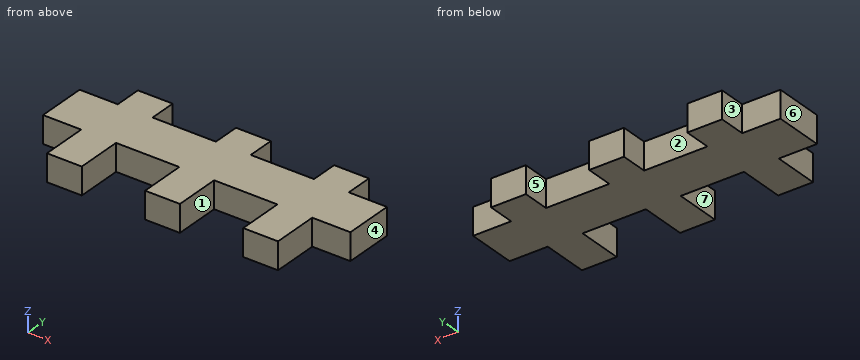
from build123d import *

# Parameters (mm, degrees)
SKETCH1_W           = 4
SKETCH1_H           = 3.175
SKETCH1_W_2         = 42.3
SKETCH1_H_2         = 5.7
SKETCH1_H_3         = 2.225
BOSS_EXTRUDE1_DEPTH = 3.175
CUT_EXTRUDE2_DEPTH  = 23.175
BOSS_EXTRUDE2_DEPTH = 3.175


with BuildPart() as part:
    # Sketch1 → Boss-Extrude1 (new body)
    with BuildSketch(Plane.XY):
        with Locations((-11.5, -1.5875)):
            Rectangle(SKETCH1_W, SKETCH1_H)
        with Locations((-11.5, 7.2875)):
            Rectangle(SKETCH1_W, SKETCH1_H)
        with Locations((0, 7.2875)):
            Rectangle(SKETCH1_W, SKETCH1_H)
        with Locations((0, -1.5875)):
            Rectangle(SKETCH1_W, SKETCH1_H)
        with Locations((11.5, 7.2875)):
            Rectangle(SKETCH1_W, SKETCH1_H)
        with Locations((11.5, -1.5875)):
            Rectangle(SKETCH1_W, SKETCH1_H)
        with Locations((0, 2.85)):
            Rectangle(SKETCH1_W_2, SKETCH1_H_2)
        with Locations((-11.5, -4.2875)):
            Rectangle(SKETCH1_W, SKETCH1_H_3)
        with Locations((0, -4.2875)):
            Rectangle(SKETCH1_W, SKETCH1_H_3)
        with Locations((11.5, -4.2875)):
            Rectangle(SKETCH1_W, SKETCH1_H_3)
    extrude(amount=BOSS_EXTRUDE1_DEPTH)

    # Sketch2 → Cut-Extrude2 (cut)
    with BuildSketch(Plane(origin=(0, 5.7, 0), x_dir=(1, 0, 0), z_dir=(0, 1, 0))):
        Polygon((-17.975, 0), (-21.15, 0), (-21.15, -3.175), align=None)
        Polygon((-17.975, -3.175), (-17.975, 0), (-21.15, -3.175), align=None)
        Polygon((21.15, -3.175), (17.975, -3.175), (17.975, 0), align=None)
        Polygon((21.15, -3.175), (17.975, 0), (21.15, 0), align=None)
    extrude(amount=-CUT_EXTRUDE2_DEPTH, mode=Mode.SUBTRACT)

    # Sketch3 → Boss-Extrude2 (add)
    with BuildSketch(Plane.XY.offset(3.175)):
        Polygon((-13.54064, -5.44064), (-9.45936, -5.44064), (-9.45936, -0.04064), (-2.04064, -0.04064), (-2.04064, -5.44064), (2.04064, -5.44064), (2.04064, -0.04064), (9.45936, -0.04064), (9.45936, -5.44064), (13.54064, -5.44064), (13.54064, -0.04064), (18.01564, -0.04064), (18.01564, 5.74064), (13.54064, 5.74064), (13.54064, 8.91564), (9.45936, 8.91564), (9.45936, 5.74064), (2.04064, 5.74064), (2.04064, 8.91564), (-2.04064, 8.91564), (-2.04064, 5.74064), (-9.45936, 5.74064), (-9.45936, 8.91564), (-13.54064, 8.91564), (-13.54064, 5.74064), (-18.01564, 5.74064), (-18.01564, -0.04064), (-13.54064, -0.04064), align=None)
    extrude(amount=-BOSS_EXTRUDE2_DEPTH)


solid = part.part
Read the model definition and answer for the solid it produces. Units are mm, in the model's axes. Face numbers are marked on the shaded views. A direction names the side the tool comes from. Round coordinates to 2 decimals unless told otherwise and drop trailing zeros. Write each loop counter-clockwise with the first axis right and the second up, starting at its lowest first coordinate (ties: lowest second). Pieces come first, ordered by that corner, then holes. Notation, with made-up numbers: (-6, 27.5) - (19, 27.5) arc R26 cw to (19, 48.5) - close; hole circle Ø4 at (48, 15). An arc over 180 degrees is marked (long way). Use a Markdown table: item, result.
(1) Each of these flat-tipped pins is pushed along its axis until it touches: pin 1 Ø1 at (x, z) = (7.5, 1) entering from -Y; pin 2 Ø1.6 at (y, z) = (-2.5, 2.5) entering from -X; pin 3 Ø1 at (y, z) = (-3, 2.5) entering from +X; pin 4 Ø2 at (x, y) = (12.5, -3) entering from -Z. Where does it stop, or does it pass through?
Reported:
| item | result |
|---|---|
| pin 1 | y = -0.04 |
| pin 2 | x = -13.54 |
| pin 3 | x = 13.54 |
| pin 4 | z = 0 |
(2) The mould has two halves that part along X. Classify the marked faces 4, 5, 6 and 7: released by +X, released by -X, zero draft, split by the parting line, or undercut.
Reported:
| item | result |
|---|---|
| face 4 | released by +X |
| face 5 | undercut |
| face 6 | released by -X |
| face 7 | undercut |
(3) Straight lines are drawn through the part: line 1 along X through (y, z) = (8, 1.95); line 2 along Y through (x, z) = (-4, 2.15). For each, find the intervals that lie inside material, in ascending order. Write a range as [from, to].
Reported:
| item | result |
|---|---|
| line 1 | [-13.54, -9.46], [-2.04, 2.04], [9.46, 13.54] |
| line 2 | [-0.04, 5.74] |
(4) The part is cut by section A-A (z = 1.45). Write down the section's boundary in (x, y), then the cut area to 3 significant figures.
Reported:
| item | result |
|---|---|
| outline | (-18.02, -0.04) - (-13.54, -0.04) - (-13.54, -5.44) - (-9.46, -5.44) - (-9.46, -0.04) - (-2.04, -0.04) - (-2.04, -5.44) - (2.04, -5.44) - (2.04, -0.04) - (9.46, -0.04) - (9.46, -5.44) - (13.54, -5.44) - (13.54, -0.04) - (18.02, -0.04) - (18.02, 5.74) - (13.54, 5.74) - (13.54, 8.92) - (9.46, 8.92) - (9.46, 5.74) - (2.04, 5.74) - (2.04, 8.92) - (-2.04, 8.92) - (-2.04, 5.74) - (-9.46, 5.74) - (-9.46, 8.92) - (-13.54, 8.92) - (-13.54, 5.74) - (-18.02, 5.74) - close |
| area | 313 mm2 |
(5) The part is cut by section B-B (y = -4). Write down the section's boundary in (x, z) (3 decimals), then the cut area to 3 significant figures.
Reported:
| item | result |
|---|---|
| outline | (-13.541, 0) - (-9.459, 0) - (-9.459, 3.175) - (-13.541, 3.175) - close; (-2.041, 0) - (2.041, 0) - (2.041, 3.175) - (-2.041, 3.175) - close; (9.459, 0) - (13.541, 0) - (13.541, 3.175) - (9.459, 3.175) - close |
| area | 38.9 mm2 |
(6) Which of the six approach directions +Z, -Z, +X, -X, +Y, -Y give full straight-line access (tool end or side, diameter ignored) to the marked faces 1, 2 and 3?
Reported:
| item | result |
|---|---|
| face 1 | +Z, -Z, -Y |
| face 2 | +Z, -Z, +Y |
| face 3 | +Z, -Z, -X, +Y |
(7) The part is cut by section C-C (x = -15). Write down the section's boundary in (y, z) (3 decimals), then the cut area to 3 significant figures.
Reported:
| item | result |
|---|---|
| outline | (-0.041, 0) - (5.741, 0) - (5.741, 3.175) - (-0.041, 3.175) - close |
| area | 18.4 mm2 |
